Geometry check sheet. Reference: the model listing, model coordinates, mm. Face numbers are marked on the shaded views. Give positions to 0.01 mm unless a question says otherwise; leave off trailing zeros. Loops run counter-clockwise (first coordinate to the right, second up) from the corner with the lowest first, then second, coordinate; pieces in that order, holes last. Notation, with made-up numbers: (35.25, 33.25) -> (46.25, 33.25) arc R15 cw to (46.25, 40.25) -> close; hole circle Ø3 at (5.25, 33.25). An arc over 180 degrees is marked (long way). Write each question's results on one line, items separated by ' | '. Start each with the question number.
1) Sectioned sample at A-A on z = 33. Record the cut outline in (x, y).
2) Depth check by flat-ended pin: pin 1 (5 mm diameter, centred on y = -58.5, z = 5.5, fed in from +X); pin 2 (1.6 mm diameter, centred on y = -24.5, z = 0.5, fed in from -X); pin 3 (2 mm diameter, centred on y = -19, z = 0.5, fed in from -X). Enter the tip coordinate at first touch or a pass-through.
3) Draft check along X on the marked faces 1 and 2. Enter one of: pulls with the +X half, pulls with the -X half, needs draft (parallel to the pull), parting line crosses it, or undercut.
4) Scan lines: line 1 (X direction, y = -60.5, z = 9.5); line 2 (Z direction, x = -5, y = -62); line 3 (Z direction, x = -4.5, y = -32). Record each from-to range of solid material in increasing order. Write a range as from..to.
5) Sectioned sample at B-B on y = 3.5. Count the separate pieces of the cut face and the enclosed holes in it, then the cut area to 3 significant figures.
```python
from build123d import *

# Parameters (mm, degrees)
F1_DEPTH = 2
F3_DEPTH = 17.200789751
F4_W     = 1
F4_H     = 2
F5_DEPTH = 25
F7_DEPTH = 2
F9_DEPTH = 0.2


# Not quite as in the source:
# - the dataset's text gives a spline's control points without its knots; the knots are read off the source's solid
# - a feature names something its author has since deleted; it is built from what else it names


with BuildPart() as f1:
    # F0 (on Top) → F1 (new body)
    with BuildSketch(Plane.XY):
        with BuildLine():
            ThreePointArc((6.4629719502, -7.6308579839), (9.0727537028, -4.2053704057), (10, 0))
            ThreePointArc((10, 0), (-5.9694275413, 8.0228383275), (-2.8731869657, -9.5783504143))
            Line((-2.8731869657, -9.5783504143), (0, 0))
            Line((0, 0), (1.8618540828, -6.2738101865))
            add(Edge.make_bspline(
                [(1.8618540828, -6.2738101865), (1.9794198127, -6.3341629295), (2.5732776532, -6.6333178765), (3.6057370778, -7.0964112527), (4.8687885055, -7.50576435), (5.8045739388, -7.6494945297), (6.2976751035, -7.6438504545), (6.4629719502, -7.6308579839)],
                knots=[0.0471973375, 0.0471973375, 0.0471973375, 0.0471973375, 0.0625, 0.125, 0.1875, 0.25, 0.2838293075, 0.2838293075, 0.2838293075, 0.2838293075], degree=3))
        make_face()
        with BuildLine():
            Line((0, 0), (-2.8731869657, -9.5783504143))
            ThreePointArc((-2.8731869657, -9.5783504143), (-0.0146952719, -9.9999892024), (2.8450232941, -9.5867534888))
            Line((2.8450232941, -9.5867534888), (2.4577875555, -8.2819017585))
            Line((2.4577875555, -8.2819017585), (1.8618540828, -6.2738101865))
            Line((1.8618540828, -6.2738101865), (0, 0))
        make_face()
        with BuildLine():
            ThreePointArc((2.8450232941, -9.5867534888), (-0.0146952719, -9.9999892024), (-2.8731869657, -9.5783504143))
            Line((-2.8731869657, -9.5783504143), (-3.241058439, -10.8047244445))
            Line((-3.241058439, -10.8047244445), (3.2064757654, -10.8047244445))
            Line((3.2064757654, -10.8047244445), (2.8450232941, -9.5867534888))
        make_face()
        with BuildLine():
            add(Edge.make_bspline(
                [(6.4629719502, -7.6308579839), (6.6030627596, -7.619846729), (6.8840296576, -7.5803052276), (7.2792450589, -7.4693493545), (7.6665868261, -7.2958798164), (8.0522350381, -7.0483493763), (8.4601010219, -6.700195356), (8.8775961576, -6.2496121629), (9.4379128784, -5.5115962551), (10.1252991034, -4.3405271139), (10.8897039738, -2.5813381399), (11.5728725961, -0.5166619682), (12.3603130252, 2.5826938425), (13.095778184, 6.9972675513), (13.399766994, 10.8869404738), (13.4782410246, 12.8689533823)],
                knots=[0.2838293075, 0.2838293075, 0.2838293075, 0.2838293075, 0.3125, 0.34375, 0.375, 0.40625, 0.4375, 0.46875, 0.5, 0.5625, 0.625, 0.6875, 0.75, 0.875, 1, 1, 1, 1], degree=3))
            ThreePointArc((6.4629719502, -7.6308579839), (5.4847517485, -8.3616683896), (4.4247539743, -8.9678064356))
            add(Edge.make_bspline(
                [(4.4247539743, -8.9678064356), (5.941531364, -9.347351876), (11.7155314673, -9.1561084525), (14.6416607546, 2.8636422945), (15.0353610516, 12.807302177)],
                knots=[0.1854268528, 0.1854268528, 0.1854268528, 0.1854268528, 0.3850411547, 1, 1, 1, 1], degree=3))
            Line((15.0353610516, 12.807302177), (13.4782410246, 12.8689533823))
        make_face()
        with BuildLine():
            ThreePointArc((4.4247539743, -8.9678064356), (5.4847517485, -8.3616683896), (6.4629719502, -7.6308579839))
            add(Edge.make_bspline(
                [(1.8618540828, -6.2738101865), (1.9794198127, -6.3341629295), (2.5732776532, -6.6333178765), (3.6057370778, -7.0964112527), (4.8687885055, -7.50576435), (5.8045739388, -7.6494945297), (6.2976751035, -7.6438504545), (6.4629719502, -7.6308579839)],
                knots=[0.0471973375, 0.0471973375, 0.0471973375, 0.0471973375, 0.0625, 0.125, 0.1875, 0.25, 0.2838293075, 0.2838293075, 0.2838293075, 0.2838293075], degree=3))
            Line((1.8618540828, -6.2738101865), (2.4577875555, -8.2819017585))
            add(Edge.make_bspline(
                [(2.4577875555, -8.2819017585), (3.1280804798, -8.5721149462), (3.7854626045, -8.8078356145), (4.4247539743, -8.9678064356)],
                knots=[0.1012934121, 0.1012934121, 0.1012934121, 0.1012934121, 0.1854268528, 0.1854268528, 0.1854268528, 0.1854268528], degree=3))
        make_face()
        with BuildLine():
            Line((2.4577875555, -8.2819017585), (2.8450232941, -9.5867534888))
            ThreePointArc((2.8450232941, -9.5867534888), (3.6480390961, -9.3108437186), (4.4247539743, -8.9678064356))
            add(Edge.make_bspline(
                [(2.4577875555, -8.2819017585), (3.1280804798, -8.5721149462), (3.7854626045, -8.8078356145), (4.4247539743, -8.9678064356)],
                knots=[0.1012934121, 0.1012934121, 0.1012934121, 0.1012934121, 0.1854268528, 0.1854268528, 0.1854268528, 0.1854268528], degree=3))
        make_face()
        Polygon((3.2064757654, -10.8047244445), (-3.241058439, -10.8047244445), (-8.6003948755, -10.8047244445), (-8.6003948755, -15.9862233672), (-8.6003948755, -17.2114234168), (-7.6003948755, -17.2114234168), (-7.6003948755, -20.2114234168), (-8.6003948755, -20.2114234168), (-8.6003948755, -23.9146029156), (-7.6003948755, -23.9146029156), (-7.6003948755, -26.9146029156), (-8.6003948755, -26.9146029156), (-8.6003948755, -40.0244813867), (8.6003948755, -40.0244813867), (8.6003948755, -26.9146029156), (7.6003948755, -26.9146029156), (7.6003948755, -23.9146029156), (8.6003948755, -23.9146029156), (8.6003948755, -20.2114234168), (7.6003948755, -20.2114234168), (7.6003948755, -17.2114234168), (8.6003948755, -17.2114234168), (8.6003948755, -15.9862233672), (8.6003948755, -10.8047244445), align=None)
        Polygon((-8.6003948755, -15.9862233672), (-8.6003948755, -10.8047244445), (-11.7467804993, -13.3954739058), align=None)
        with BuildLine():
            Line((-11.7467804993, -13.3954739058), (-8.6003948755, -10.8047244445))
            Line((-8.6003948755, -10.8047244445), (-17.2348651583, -3.6950589713))
            Line((-17.2348651583, -3.6950589713), (-10.8148216824, 7.9533712388))
            ThreePointArc((-10.8148216824, 7.9533712388), (-11.6010166189, 10.6703360015), (-14.3179813816, 9.884141065))
            Line((-14.3179813816, 9.884141065), (-21.7172442848, -3.5409701289))
            Line((-21.7172442848, -3.5409701289), (-21.7148243129, -5.1877374014))
            Line((-21.7148243129, -5.1877374014), (-11.7467804993, -13.3954739058))
        make_face()
        with BuildLine():
            Line((21.7148243129, -21.6032104103), (8.6003948755, -10.8047244445))
            Line((8.6003948755, -10.8047244445), (8.6003948755, -15.9862233672))
            Line((8.6003948755, -15.9862233672), (17.2348651583, -23.0958888404))
            Line((17.2348651583, -23.0958888404), (10.8148216824, -34.7443190505))
            ThreePointArc((10.8148216824, -34.7443190505), (11.6010166189, -37.4612838132), (14.3179813816, -36.6750888767))
            Line((14.3179813816, -36.6750888767), (21.7172442848, -23.2499776828))
            Line((21.7172442848, -23.2499776828), (21.7148243129, -21.6032104103))
        make_face()
    extrude(amount=F1_DEPTH)

    # F2 (on face) → F3 (join, through all)
    with BuildSketch(Plane.YZ.offset(8.6003948755)):
        Polygon((-40.0244813867, 0), (-40.0244813867, 2), (-66.176410403, 12.9284200062), (-66.8879257534, 11.2257494531), align=None)
        Polygon((-66.8879257534, 11.2257494531), (-66.176410403, 12.9284200062), (-68.0217670369, 13.6995612992), (-68.7332823873, 11.9968907461), align=None)
        Polygon((-68.0217670369, 13.6995612992), (-66.176410403, 12.9284200062), (-63.8033605813, 18.6071759886), (-65.6487172152, 19.3783172816), align=None)
    extrude(amount=-F3_DEPTH)

    # F4 (on face) → F5 (cut)
    with BuildSketch(Plane(origin=(0, -2.8656632843, -6.8575899128), x_dir=(1, 0, 0), z_dir=(0, 0.3855706465, 0.9226783169))):
        with Locations((-0.5, -67.044358232)):
            Rectangle(F4_W, F4_H)
        with BuildLine():
            Line((1, -68.044358232), (0, -68.044358232))
            Line((0, -68.044358232), (-1, -68.044358232))
            Line((-1, -68.044358232), (-1, -69.7565637529))
            ThreePointArc((-1, -69.7565637529), (0, -70.7565637529), (1, -69.7565637529))
            Line((1, -69.7565637529), (1, -68.044358232))
        make_face()
        with Locations((0.5, -67.044358232)):
            Rectangle(F4_W, F4_H)
        with BuildLine():
            Line((-1, -66.044358232), (0, -66.044358232))
            Line((0, -66.044358232), (1, -66.044358232))
            Line((1, -66.044358232), (1, -44.7565637529))
            ThreePointArc((1, -44.7565637529), (0, -43.7565637529), (-1, -44.7565637529))
            Line((-1, -44.7565637529), (-1, -66.044358232))
        make_face()
    extrude(amount=-F5_DEPTH, mode=Mode.SUBTRACT)

    # F6 (on face) → F7 (join)
    with BuildSketch(Plane(origin=(0, -62.7830539309, 26.2359071944), x_dir=(1, 0, 0), z_dir=(0, -0.9226783169, 0.3855706465))):
        with BuildLine():
            ThreePointArc((-1.8515158445, 14.0382554382), (-8.3589539863, 15.7649961788), (-14.8663921282, 14.0382554382))
            Line((-14.8663921282, 14.0382554382), (-1.8515158445, 14.0382554382))
        make_face()
        Polygon((1, -15.4322651642), (8.6003948755, -15.4322651642), (8.6003948755, -14.2483813688), (8.6003948755, -7.4322651642), (1, -7.4322651642), align=None)
        with BuildLine():
            Line((8.6003948755, -7.4322651642), (8.6003948755, -14.2483813688))
            Line((8.6003948755, -14.2483813688), (14.8663921282, 14.0382554382))
            ThreePointArc((14.8663921282, 14.0382554382), (8.3589539863, 15.7649961788), (1.8515158445, 14.0382554382))
            Line((1.8515158445, 14.0382554382), (1, -7.4322651642))
            Line((1, -7.4322651642), (8.6003948755, -7.4322651642))
        make_face()
        Polygon((-8.6003948755, -7.4322651642), (-1, -7.4322651642), (-1.8515158445, 14.0382554382), (-14.8663921282, 14.0382554382), (-8.6003948755, -14.2483813688), align=None)
    extrude(amount=-F7_DEPTH)

    # F8 (on face) → F9 (join)
    with BuildSketch(Plane.XY.offset(2)):
        with BuildLine():
            Line((8.3395420131, 5.5183366165), (-8.3395420131, 5.5183366165))
            ThreePointArc((-8.3395420131, 5.5183366165), (-9.6548741312, 2.6044971704), (-9.9834241522, -0.575536443))
            Line((-9.9834241522, -0.575536443), (-8.1826943192, -3.206660389))
            Line((-8.1826943192, -3.206660389), (-1.5899471466, -3.206660389))
            Line((-1.5899471466, -3.206660389), (0, -0.575536443))
            Line((0, -0.575536443), (1.5899471466, -3.206660389))
            Line((1.5899471466, -3.206660389), (8.1826943192, -3.206660389))
            Line((8.1826943192, -3.206660389), (9.9834241522, -0.575536443))
            ThreePointArc((9.9834241522, -0.575536443), (9.6548741312, 2.6044971704), (8.3395420131, 5.5183366165))
        make_face()
        with BuildLine():
            ThreePointArc((-8.9966146265, -0.2468304304), (-8.721852762, 2.2201991799), (-7.7836131854, 4.5183366165))
            Line((-7.7836131854, 4.5183366165), (7.7836131854, 4.5183366165))
            ThreePointArc((7.7836131854, 4.5183366165), (8.721852762, 2.2201991799), (8.9966146265, -0.2468304304))
            Line((8.9966146265, -0.2468304304), (7.6553154911, -2.206660389))
            Line((7.6553154911, -2.206660389), (2.1540632086, -2.206660389))
            Line((2.1540632086, -2.206660389), (0, 1.3579909904))
            Line((0, 1.3579909904), (-2.1540632086, -2.206660389))
            Line((-2.1540632086, -2.206660389), (-7.6553154911, -2.206660389))
            Line((-7.6553154911, -2.206660389), (-8.9966146265, -0.2468304304))
        make_face(mode=Mode.SUBTRACT)
    extrude(amount=F9_DEPTH)


solid = f1.part
```
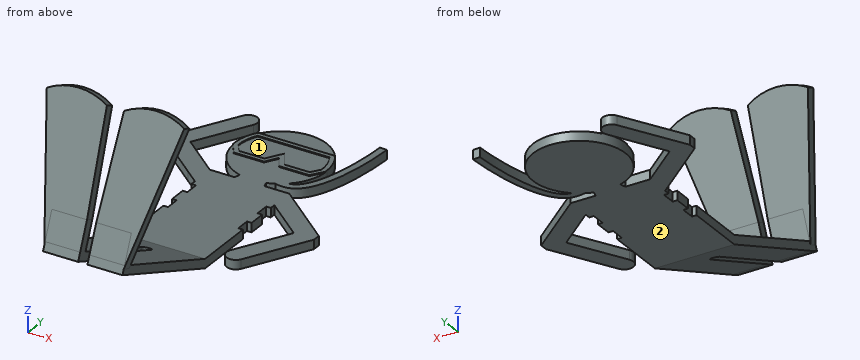
Result:
1) outline: (-13.57, -57.79) -> (-13.38, -59.96) -> (-1.59, -59.96) -> (-1.62, -57.79) -> close; (1.59, -59.96) -> (13.38, -59.96) -> (13.57, -57.79) -> (1.62, -57.79) -> close
2) pin 1: x = 8.6 | pin 2: x = -8.6 | pin 3: x = -7.6
3) face 1: undercut | face 2: needs draft
4) line 1: -8.6..-1, 1..8.6 | line 2: 9.18..11.18, 22.92..28.11 | line 3: 0..2
5) separate pieces: 3 | enclosed holes: 0 | area: 50.2 mm^2
